Design review of the part built by this model. Coordinates are the model's own, in mm. A direction names the side the tool comes from. Give positions to 0.01 mm unless a question says otherwise; leave off trailing zeros. Write each question's results on one line, items separated by ' | '. Start each with the question number.
(1) To check wall thickness, follow probe 1 along Z at (x, y) = (48.5, 5); probe 2 along Z at (x, y) = (31.5, 7.25); probe 3 along Z at (x, y) = (31, 9.75). State the ranges of each line that lie inside material, in increasing order.
(2) Take a section at A-A (y = 4). Count the separate pieces of the cut face and the enclosed holes in it, plus the area to 3 significant figures.
(3) For faces 4 (the face through (48.254, 24.26, 23.21)), 5 (the face through (46, 4, 10.819)), 6 (the face through (33.124, 11.586, 6.201)), 7 (the face through (31, 24, 9.569)), list the 3-axis set-ups (+Z, -Z, +X, -X, +Y, -Y) from which the entire face can be reached by the end or side of a thin tool; tool diameter is ignored.
(4) Mouldability with a two-part tool opening along X and no side actions: class faces 1 (the face through (26.76, 12.32, 4.6)), 2 (the face through (35.89, 0.93, 14.46)), 3 (the face through (38, 12, 4.319)) as released by +X, released by -X, zero draft, split by the parting line, or undercut.
(5) Clearance check with flat-ended pins moving along their axes: pin 1 (5.5 mm diameter, centred on x = 38.46, y = 4, fed in from -Z); pin 2 (1.6 mm diameter, centred on x = 31, y = 24.5, fed in from -Z). State where each tip first meets the part, or that it passes through.
from build123d import *

# Parameters (mm, degrees)
CROQUIS1_W              = 23.999999999999773
CROQUIS1_H              = 19.99999938803319
SALIENTE_EXTRUIR1_DEPTH = 25
CORTAR_EXTRUIR1_DEPTH   = 60.75663166018996
CROQUIS3_R              = 5.599999999999993
CORTAR_EXTRUIR2_DEPTH   = 43.33702219441687
CROQUIS4_R              = 1.6999999999999995
CORTAR_EXTRUIR3_DEPTH   = 62.33741517329244
CROQUIS8_W              = 7.000000000000005
CROQUIS8_H              = 2.499999999999975
CORTAR_EXTRUIR7_DEPTH   = 1.5
REDONDEO1_R             = 1


with BuildPart() as part:
    # Croquis1 → Saliente-Extruir1 (new body)
    with BuildSketch(Plane.XZ):
        with Locations((38.456466898211374, 14.319199476403412)):
            Rectangle(CROQUIS1_W, CROQUIS1_H)
    extrude(amount=-SALIENTE_EXTRUIR1_DEPTH)

    # Croquis2 → Cortar-Extruir1 (cut, through all)
    with BuildSketch(Plane.XY.offset(24.319199170420006)):
        with BuildLine():
            Line((35.456466898211275, 0), (36.335146554651615, 1.8786796564403407))
            ThreePointArc((36.335146554651615, 1.8786796564403407), (38.45646689821126, 7.00000000000005), (40.57778724177091, 1.8786796564403407))
            Line((40.57778724177091, 1.8786796564403407), (41.45646689821126, 0))
            Line((41.45646689821126, 0), (35.456466898211275, 0))
        make_face()
    extrude(amount=-CORTAR_EXTRUIR1_DEPTH, mode=Mode.SUBTRACT)

    # Croquis3 → Cortar-Extruir2 (cut, through all)
    with BuildSketch(Plane(origin=(50.45646689821126, 0, 0), x_dir=(0, 0, -1), z_dir=(1, 0, 0))):
        with Locations((-14.319199170420013, 17.499998559923498)):
            Circle(CROQUIS3_R)
    extrude(amount=-CORTAR_EXTRUIR2_DEPTH, mode=Mode.SUBTRACT)

    # Croquis4 → Cortar-Extruir3 (cut, through all)
    with BuildSketch(Plane.XZ):
        with Locations(Location((31.464341614174252, 22.06919978238682, 0), (0, 0, 270))):
            Circle(CROQUIS4_R)
        with Locations(Location((45.448592182248724, 22.06919978238682, 0), (0, 0, 90))):
            Circle(CROQUIS4_R)
        with Locations(Location((45.448592182248724, 6.5691985584531984, 0), (0, 0, 270))):
            Circle(CROQUIS4_R)
        with Locations(Location((31.464341614174252, 6.569198558453197, 0), (0, 0, 90))):
            Circle(CROQUIS4_R)
    extrude(amount=-CORTAR_EXTRUIR3_DEPTH, mode=Mode.SUBTRACT)

    # Cortar-Barrer2: sweep along a path in Croquis9
    with BuildLine(Plane(origin=(0, 0, 10.819199782386816), x_dir=(-1, 0, 0), z_dir=(0, 0, -1))) as cortar_barrer2_path:
        Line((-50.45646689821126, 6.999998762857437), (-48.45646689821129, 6.999998762857437))
        ThreePointArc((-48.45646689821129, 6.999998762857437), (-44.92093299227851, 5.5355326687901805), (-43.45646689821125, 1.9999987628574059))
        Line((-43.45646689821125, 1.9999987628574059), (-43.45646689821125, -1.23714255593e-06))
    # Croquis8 → Cortar-Barrer2 (sweep, cut)
    with BuildSketch(Plane(origin=(50.45646689821126, 0, 0), x_dir=(0, 0, -1), z_dir=(1, 0, 0))):
        with Locations((-14.319199782386818, 5.749998762857451)):
            Rectangle(CROQUIS8_W, CROQUIS8_H)
    cortar_barrer2 = sweep(path=cortar_barrer2_path.line, mode=Mode.SUBTRACT)

    # Simetría1: Cortar-Barrer2 across plane
    add(cortar_barrer2.mirror(Plane(origin=(38.45646689821126, 0, 0), x_dir=(0, 0, 1), z_dir=(1, 0, 0))), mode=Mode.SUBTRACT)

    # Croquis11 → Cortar-Extruir7 (cut)
    with BuildSketch(Plane(origin=(0, 25, 0), x_dir=(1, 0, 0), z_dir=(0, 1, 0))):
        Polygon((47.180642989817585, -19.069199782386846), (43.716541374679856, -19.069199782386846), (41.98449056711099, -22.06919978238682), (43.716541374679856, -25.0691997823868), (47.180642989817585, -25.0691997823868), (48.91269379738645, -22.06919978238682), align=None)
        Polygon((34.928443229312, -22.06919978238682), (33.196392421743134, -19.069199782386825), (29.732290806605373, -19.069199782386825), (28.000239999036502, -22.06919978238682), (29.73229080660538, -25.069199782386818), (33.19639242174313, -25.069199782386814), align=None)
        Polygon((34.928443229312016, -6.569198558453194), (33.196392421743134, -3.569198558453189), (29.732290806605366, -3.56919855845319), (28.000239999036484, -6.569198558453203), (29.732290806605363, -9.569198558453209), (33.196392421743134, -9.569198558453209), align=None)
        Polygon((47.18064298981763, -9.569198558453236), (48.91269379738652, -6.569198558453209), (47.18064298981762, -3.5691985584531754), (43.716541374679835, -3.5691985584531754), (41.98449056711095, -6.569198558453195), (43.71654137467985, -9.569198558453236), align=None)
    extrude(amount=-CORTAR_EXTRUIR7_DEPTH, mode=Mode.SUBTRACT)

    # Redondeo1
    # the kernel refuses this fillet: 1 mm, written as the material it takes off along each edge
    with BuildSketch(Plane(origin=(50.45646689821126, 25, 26.819199170420006), x_dir=(0, -1, 0), z_dir=(0, 0, -1))) as redondeo1_piece_1:
        with BuildLine():
            CenterArc((REDONDEO1_R, REDONDEO1_R), REDONDEO1_R, 180, 90)
            Line((0, REDONDEO1_R), (0, 0))
            Line((0, 0), (REDONDEO1_R, 0))
        make_face()
    extrude(amount=24.99999938803319, mode=Mode.SUBTRACT)
    with BuildSketch(Plane(origin=(38.45646689821127, 4.000000000000019, 4.319199782386818), x_dir=(0.003141587485877974, -0.9999950652018582, 0), z_dir=(-0.9999950652018582, -0.003141587485877974, 0))) as redondeo1_piece_2:
        with BuildLine():
            CenterArc((3.0000000000000306 + REDONDEO1_R, REDONDEO1_R), REDONDEO1_R, 180, 90)
            Line((3.0000000000000306 + REDONDEO1_R, 0), (3.0000000000000306, 0))
            Line((3.0000000000000306, 0), (3.0000000000000306, REDONDEO1_R))
        make_face()
    revolve(axis=Axis((38.45646689821127, 4.000000000000019, 4.319199782386818), (0, 0, 1)), revolution_arc=359.64, mode=Mode.SUBTRACT)
    with BuildSketch(Plane(origin=(38.45646689821127, 4.000000000000019, 24.319199170420006), x_dir=(-0.0031415874858803424, -0.9999950652018582, 0), z_dir=(0.9999950652018582, -0.0031415874858803424, 0))) as redondeo1_piece_3:
        with BuildLine():
            CenterArc((3.0000000000000298 + REDONDEO1_R, REDONDEO1_R), REDONDEO1_R, 180, 90)
            Line((3.0000000000000298, REDONDEO1_R), (3.0000000000000298, 0))
            Line((3.0000000000000298, 0), (3.0000000000000298 + REDONDEO1_R, 0))
        make_face()
    revolve(axis=Axis((38.45646689821127, 4.000000000000019, 24.319199170420006), (0, 0, -1)), revolution_arc=359.64000000000004, mode=Mode.SUBTRACT)
    with BuildSketch(Plane(origin=(26.456466898211488, 17.499998559923498, 14.319199170420013), x_dir=(0, 0, -1), z_dir=(0, -1, 0))) as redondeo1_piece_4:
        with BuildLine():
            CenterArc((5.599999999999994 + REDONDEO1_R, REDONDEO1_R), REDONDEO1_R, 180, 90)
            Line((5.599999999999994, REDONDEO1_R), (5.599999999999994, 0))
            Line((5.599999999999994, 0), (5.599999999999994 + REDONDEO1_R, 0))
        make_face()
    revolve(axis=Axis((26.456466898211488, 17.499998559923498, 14.319199170420013), (1, 0, 0)), mode=Mode.SUBTRACT)
    with BuildSketch(Plane(origin=(50.45646689821126, 17.499998559923498, 14.319199170420013), x_dir=(0, 0, -1), z_dir=(0, -1, 0))) as redondeo1_piece_5:
        with BuildLine():
            CenterArc((5.599999999999994 + REDONDEO1_R, -REDONDEO1_R), REDONDEO1_R, 90, 90)
            Line((5.599999999999994, -REDONDEO1_R), (5.599999999999994, 0))
            Line((5.599999999999994, 0), (5.599999999999994 + REDONDEO1_R, 0))
        make_face()
    revolve(axis=Axis((50.45646689821126, 17.499998559923498, 14.319199170420013), (1, 0, 0)), mode=Mode.SUBTRACT)
    with BuildSketch(Plane(origin=(26.456466898211488, 25, 1.8191997823868178), x_dir=(1, 0, 0), z_dir=(0, 0, 1))) as redondeo1_piece_6:
        with BuildLine():
            CenterArc((REDONDEO1_R, -REDONDEO1_R), REDONDEO1_R, 90, 90)
            Line((0, -REDONDEO1_R), (0, 0))
            Line((0, 0), (REDONDEO1_R, 0))
        make_face()
    extrude(amount=24.99999938803319, mode=Mode.SUBTRACT)
    with BuildSketch(Plane(origin=(26.456466898211488, -2.5, 24.319199170420006), x_dir=(1, 0, 0), z_dir=(0, 1, 0))) as redondeo1_piece_7:
        with BuildLine():
            CenterArc((REDONDEO1_R, REDONDEO1_R), REDONDEO1_R, 180, 90)
            Line((0, REDONDEO1_R), (0, 0))
            Line((0, 0), (REDONDEO1_R, 0))
        make_face()
    extrude(amount=30.000000000000004, mode=Mode.SUBTRACT)
    with BuildSketch(Plane(origin=(50.45646689821126, -2.5, 24.319199170420006), x_dir=(-1, 0, 0), z_dir=(0, 1, 0))) as redondeo1_piece_8:
        with BuildLine():
            CenterArc((REDONDEO1_R, -REDONDEO1_R), REDONDEO1_R, 90, 90)
            Line((0, -REDONDEO1_R), (0, 0))
            Line((0, 0), (REDONDEO1_R, 0))
        make_face()
    extrude(amount=30.000000000000004, mode=Mode.SUBTRACT)
    with BuildSketch(Plane(origin=(50.45646689821126, -2.5, 4.319199782386818), x_dir=(0, 0, 1), z_dir=(0, 1, 0))) as redondeo1_piece_9:
        with BuildLine():
            CenterArc((REDONDEO1_R, -REDONDEO1_R), REDONDEO1_R, 90, 90)
            Line((0, -REDONDEO1_R), (0, 0))
            Line((0, 0), (REDONDEO1_R, 0))
        make_face()
    extrude(amount=30.000000000000004, mode=Mode.SUBTRACT)
    with BuildSketch(Plane(origin=(26.456466898211488, -2.5, 4.319199782386818), x_dir=(0, 0, 1), z_dir=(0, 1, 0))) as redondeo1_piece_10:
        with BuildLine():
            CenterArc((REDONDEO1_R, REDONDEO1_R), REDONDEO1_R, 180, 90)
            Line((0, REDONDEO1_R), (0, 0))
            Line((0, 0), (REDONDEO1_R, 0))
        make_face()
    extrude(amount=30.000000000000004, mode=Mode.SUBTRACT)


solid = part.part
Report:
1) probe 1: 4.32 to 10.82, 17.82 to 24.32 | probe 2: 4.32 to 4.87, 8.27 to 20.37, 23.77 to 24.32 | probe 3: 4.32 to 4.93, 8.2 to 20.43, 23.7 to 24.32
2) separate pieces: 2 | enclosed holes: 6 | area: 279 mm2
3) face 4: +Y | face 5: none | face 6: +Y, -Y | face 7: -Z, +Y
4) face 1: released by -X | face 2: undercut | face 3: zero draft
5) pin 1: through | pin 2: z = 9.57
